```python
from build123d import *

# Parameters (mm, degrees)
SKETCH1_W           = 300
SKETCH1_H           = 400
SKETCH1_R           = 11
BOSS_EXTRUDE1_DEPTH = 160
FILLET1_R           = 3


with BuildPart() as part:
    # Sketch1 → Boss-Extrude1 (new body)
    with BuildSketch(Plane.XY):
        with Locations((511.639721418, 643.529340403)):
            Rectangle(SKETCH1_W, SKETCH1_H)
        with Locations((431.639721418, 526.80715456)):
            Circle(SKETCH1_R, mode=Mode.SUBTRACT)
        with Locations((431.639721418, 606.80715456)):
            Circle(SKETCH1_R, mode=Mode.SUBTRACT)
        with Locations((431.639721418, 686.80715456)):
            Circle(SKETCH1_R, mode=Mode.SUBTRACT)
        with Locations((431.639721418, 766.80715456)):
            Circle(SKETCH1_R, mode=Mode.SUBTRACT)
        with Locations((511.639721418, 526.80715456)):
            Circle(SKETCH1_R, mode=Mode.SUBTRACT)
        with Locations((511.639721418, 606.80715456)):
            Circle(SKETCH1_R, mode=Mode.SUBTRACT)
        with Locations((511.639721418, 686.80715456)):
            Circle(SKETCH1_R, mode=Mode.SUBTRACT)
        with Locations((511.639721418, 766.80715456)):
            Circle(SKETCH1_R, mode=Mode.SUBTRACT)
        with Locations((591.639721418, 526.80715456)):
            Circle(SKETCH1_R, mode=Mode.SUBTRACT)
        with Locations((591.639721418, 606.80715456)):
            Circle(SKETCH1_R, mode=Mode.SUBTRACT)
        with Locations((591.639721418, 686.80715456)):
            Circle(SKETCH1_R, mode=Mode.SUBTRACT)
        with Locations((591.639721418, 766.80715456)):
            Circle(SKETCH1_R, mode=Mode.SUBTRACT)
    extrude(amount=BOSS_EXTRUDE1_DEPTH)

    # Fillet1
    fillet1_edges = [part.edges().sort_by_distance(p)[0] for p in [
        (661.639721418, 643.529340403, 160),
        (511.639721418, 843.529340403, 160),
        (361.639721418, 643.529340403, 160),
        (511.639721418, 843.529340403, 0),
        (661.639721418, 643.529340403, 0),
        (511.639721418, 443.529340403, 0),
        (361.639721418, 643.529340403, 0),
        (361.639721418, 843.529340403, 80),
        (661.639721418, 843.529340403, 80),
        (661.639721418, 443.529340403, 80),
        (361.639721418, 443.529340403, 80),
        (511.639721418, 443.529340403, 160),
    ]]
    fillet(fillet1_edges, radius=FILLET1_R)


solid = part.part
```
Work out the finished part from the listing and answer in its coordinate system (mm). Give positions to 0.01 mm unless a question says otherwise; leave off trailing zeros. Order: outer loops, then holes, each group sorted by start corner. A loop starts at its lowest first (then second) coordinate and runs counter-clockwise, first axis right, second up. Notation, with made-up numbers: M -13,17 L 16,17 A25 cw 16,48 Z; hole C 67,5 d4. An arc over 180 degrees is marked long. Return JSON: item names as keys, results as strings.
1) Straight lines are drawn through the part: line 1 along Y through (x, z) = (512, 152); line 2 along X through (y, z) = (687, 139.5); line 3 along X through (y, z) = (762.5, 42). For each, find the intervals that lie inside material, in ascending order. Write a range as [from, to].
Resolved:
{"line 1": "[443.53, 515.81], [537.8, 595.81], [617.8, 675.81], [697.8, 755.81], [777.8, 843.53]", "line 2": "[361.64, 420.64], [442.64, 500.64], [522.64, 580.64], [602.64, 661.64]", "line 3": "[361.64, 421.52], [441.76, 501.52], [521.76, 581.52], [601.76, 661.64]"}
2) This flat-tipped pin is pushed along its axis until it touches: pin 1 (8 mm diameter, centred on x = 515, y = 555, fed in from -Z). Where does it stop, or does it pass through?
Resolved:
{"pin 1": "z = 0"}
3) Section A-A, the plane z = 29.5 is taken. Give the number of separate pieces and of enclosed holes in the cut face, plus the area to 3 significant figures.
Resolved:
{"separate pieces": "1", "enclosed holes": "12", "area": "115,000 mm^2"}
4) For a pull along Y with two mould halves and no side action, classify faces 1 (the flat face through (661.64, 641, 79)), 2 (the flat face through (510, 443.529, 79)), 3 (the flat face through (510, 843.529, 79)), 4 (the cylindrical face through (423, 760, 79)) as +Y half, -Y half, draft (parallel to the pull), parting line (faces both ways), or undercut.
Resolved:
{"face 1": "draft", "face 2": "-Y half", "face 3": "+Y half", "face 4": "undercut"}
5) Section C-C, the plane y = 681 is taken. Write down the section's boundary in (x, z), plus the area to 3 significant figures.
Resolved:
{"outline": "M 361.64,3 A3 ccw 364.64,0 L 422.3,0 L 422.3,160 L 364.64,160 A3 ccw 361.64,157 Z; M 440.98,0 L 502.3,0 L 502.3,160 L 440.98,160 Z; M 520.98,0 L 582.3,0 L 582.3,160 L 520.98,160 Z; M 600.98,0 L 658.64,0 A3 ccw 661.64,3 L 661.64,157 A3 ccw 658.64,160 L 600.98,160 Z", "area": "39,000 mm^2"}
6) Section B-B, the plane x = 593.5 is taken. Write down the section's boundary in (y, z), plus the area to 3 significant figures.
Resolved:
{"outline": "M 443.53,3 A3 ccw 446.53,0 L 515.97,0 L 515.97,160 L 446.53,160 A3 ccw 443.53,157 Z; M 537.65,0 L 595.97,0 L 595.97,160 L 537.65,160 Z; M 617.65,0 L 675.97,0 L 675.97,160 L 617.65,160 Z; M 697.65,0 L 755.97,0 L 755.97,160 L 697.65,160 Z; M 777.65,0 L 840.53,0 A3 ccw 843.53,3 L 843.53,157 A3 ccw 840.53,160 L 777.65,160 Z", "area": "50,100 mm^2"}
